Input: dimensioned drawing with shaded views. Units: mm. Origin: part minimum x, y, z. A direction names the side the tool comes from. Round coordinates to 2 decimals unless told otherwise and drop trailing zeros. Loops run counter-clockwise (first coordinate to the right, second up) from the corner with the lowest first, then second, coordinate; pieces in that order, holes last.
Item 1: Section query D-D on z = 5. Return loops of the section in (x, y).
Item 2: Section query A-A on x = 6. Return loops of the section in (y, z), then the cut area to 3 significant figures.
Item 3: Ray query, L1, parallel to Y at x = 13.75, z = 15.25; L2, parallel to X at y = 16, z = 16.75; L3, parallel to Z at x = 14.75, y = 3.75. Return the intervals inside material, ascending.
Item 4: Pull-direction query (X, two-part tool) for the marked faces 1, 2 and 3; classes: released by +X, released by -X, zero draft, split by the parting line, or undercut.
Item 5: Section query C-C on y = 13.75. Return loops of the section in (x, z).
Item 6: First-contact query: P1, Ø1.5, axis at y = 4, z = 16, coming from the +X side; P2, Ø7.5, axis at x = 15.5, z = 18, coming from the -Y side. Flat tips, straight axial feed; report the tip coordinate or a pass-through.
Item 7: Access query for the marked faces 4 and 5. Directions: +Z, -Z, +X, -X, +Y, -Y. A direction counts if a zero-diameter tool reaches every point of the face in a straight line with its end or side. Return the directions, or none.
Item 8: Section query B-B on z = 15. Return loops of the section in (x, y).
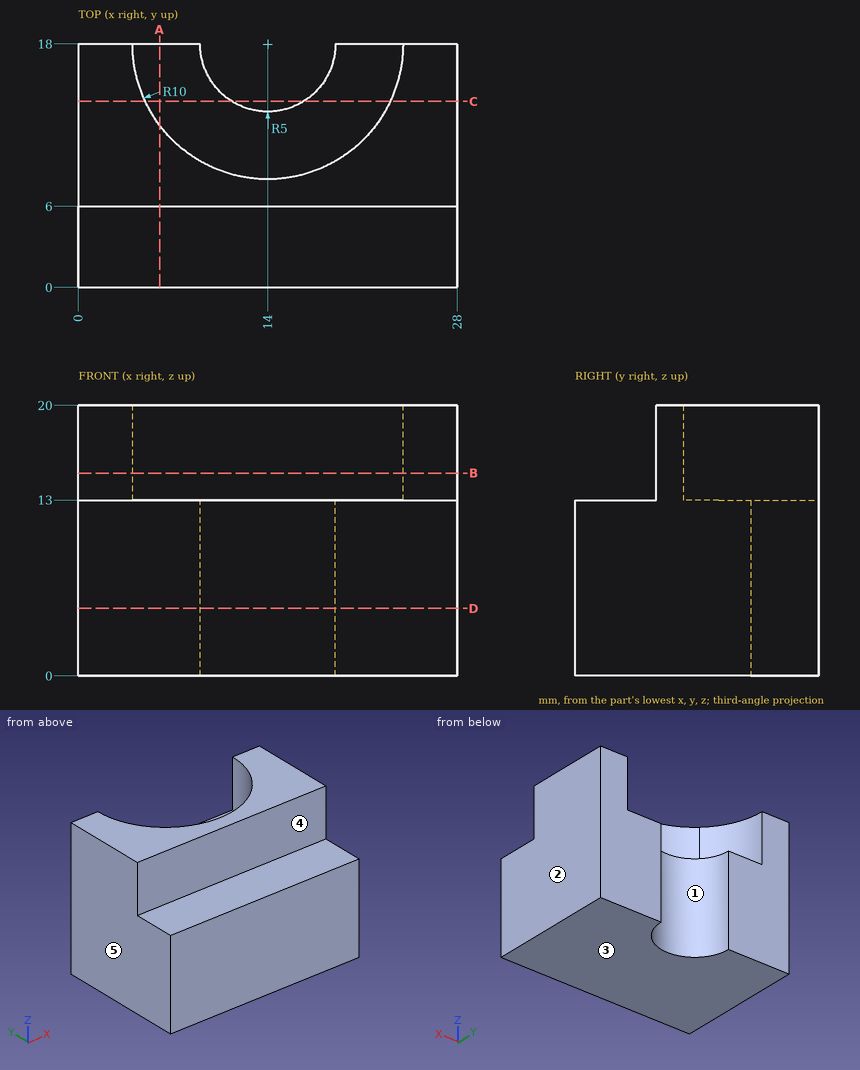
Data:
1. outline: (0, 0) - (28, 0) - (28, 18) - (19, 18) arc R5 cw to (9, 18) - (0, 18) - close
2. outline: (0, 0) - (18, 0) - (18, 13) - (12, 13) - (12, 20) - (6, 20) - (6, 13) - (0, 13) - close
2. area: 276 mm2
3. L1: y = 6 to 8
3. L2: x = 0 to 4.2, 23.8 to 28
3. L3: z = 0 to 13
4. face 1: undercut
4. face 2: released by +X
4. face 3: zero draft
5. outline: (0, 0) - (11.37, 0) - (11.37, 13) - (4.95, 13) - (4.95, 20) - (0, 20) - close; (16.63, 0) - (28, 0) - (28, 20) - (23.05, 20) - (23.05, 13) - (16.63, 13) - close
6. P1: passes through
6. P2: stops at y = 6
7. face 4: +Z, +X, -X, -Y
7. face 5: +Z, -Z, -X, +Y, -Y
8. outline: (0, 6) - (28, 6) - (28, 18) - (24, 18) arc R10 cw to (4, 18) - (0, 18) - close
